Can you work these out from the drawing? Everything is in mm from the part's minimum corner. A direction names the side the tool comes from. Coordinates: 2 decimals unless noted, no trailing zeros. Write each loop counter-clockwise with the first axis right and the second up, starting at its lowest first coordinate (ties: lowest second). Pieces come first, ordered by that corner, then holes. Notation, with made-up numbers: M -14.75,64 L -2.75,64 A15 cw -2.75,93 Z; hole C 60.5,-39 d10. An arc over 180 degrees is marked long. Write item = value, one per line.
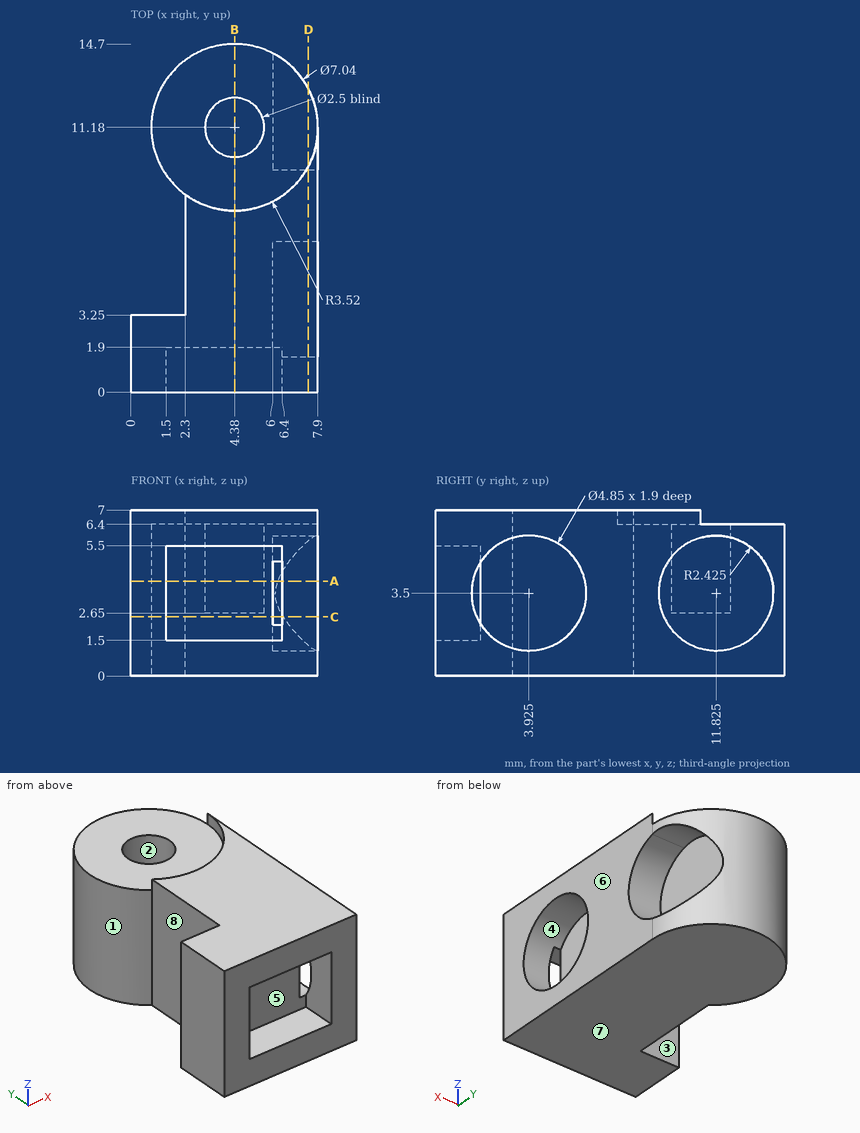
Item 1: Imagine slicing it at D-D (x = 7.5). Write out the boundary of the cut face in (y, z) (3 decimals), and give its area (3 significant figures).
Numbers:
outline = M 0,0 L 12.81,0 L 12.81,1.284 A2.425 cw long 12.81,5.716 L 12.81,6.4 L 9.55,6.4 L 9.55,7 L 0,7 Z; hole C 3.925,3.5 d4.85
area = 55.4 mm²
Item 2: Imagine slicing it at C-C (z = 2.5). Write out the boundary of the cut face in (x, y), and give its area (3 significant figures).
Numbers:
outline = M 0,0 L 1.5,0 L 1.5,1.9 L 6,1.9 L 6,6.13 L 7.9,6.13 L 7.9,9.62 L 6,9.62 L 6,14.03 L 6.44,14.03 A3.52 ccw 2.3,8.34 L 2.3,3.25 L 0,3.25 Z; M 6.4,0 L 7.9,0 L 7.9,1.72 L 6.4,1.72 Z
area = 67.6 mm²
Item 3: If we mould it in two halves opening along X, with no side actions, what happens to the marked faces 1, 2 and 3? For each: pulls with the +X half, pulls with the -X half, needs draft (parallel to the pull), parting line crosses it, or undercut.
Numbers:
face_1 = parting line crosses it
face_2 = undercut
face_3 = needs draft
Item 4: Imagine slicing it at A-A (z = 4). Write out the boundary of the cut face in (x, y), and give its area (3 significant figures).
Numbers:
outline = M 0,0 L 1.5,0 L 1.5,1.9 L 6,1.9 L 6,6.3 L 7.9,6.3 L 7.9,9.45 L 6,9.45 L 6,14.2 L 6.19,14.2 A3.52 ccw 2.3,8.34 L 2.3,3.25 L 0,3.25 Z; M 6.4,0 L 7.9,0 L 7.9,1.55 L 6.4,1.55 Z; hole C 4.38,11.18 d2.5
area = 61.8 mm²
Item 5: If I drill on line 1 along Y through (x, z) = (4.38, 4.55); line 2 along Z through (x, y) = (5, 1); line 3 along Z through (x, y) = (2, 13.25), over which ranges is the centre line in solid material (lowest first)?
Numbers:
line_1 = 1.9 to 9.93, 12.43 to 14.7
line_2 = 0 to 1.5, 5.5 to 7
line_3 = 0 to 6.4
Item 6: Imagine slicing it at B-B (x = 4.38). Write out the boundary of the cut face in (y, z), and give its area (3 significant figures).
Numbers:
outline = M 0,0 L 14.7,0 L 14.7,6.4 L 12.43,6.4 L 12.43,2.65 L 9.93,2.65 L 9.93,6.4 L 7.66,6.4 L 7.66,7 L 0,7 L 0,5.5 L 1.9,5.5 L 1.9,1.5 L 0,1.5 Z
area = 81.7 mm²
Item 7: For the marked faces 4, 5, 6, 7 and 8, which set-ups out of +Z, -Z, +X, -X, +Y, -Y let a thin tool reach every point of the face, with its end or its side?
Numbers:
face_4 = +X
face_5 = -Y
face_6 = +Z, -Z, +X, +Y, -Y
face_7 = -Z, +X, -X, +Y, -Y
face_8 = +Z, -Z, -X
Item 8: I'm going to push flat-ended pins straight in: P1, Ø1.5, axis at y = 7, z = 5, coming from the -X side; P2, Ø1, axis at x = 2, z = 1, coming from the +Y side; P3, Ø1.3, axis at y = 3.5, z = 3.5, coming from the +X side. Where does each tip first touch, or does it pass through?
Numbers:
P1 = 2.3
P2 = 14.16
P3 = 6
